Verification items for the finished model (mm, model axes). Face numbers are marked on the shaded views. A direction names the side the tool comes from. Coordinates: 2 decimals unless noted, no trailing zeros. Loops run counter-clockwise (first coordinate to the right, second up) from the corner with the lowest first, then second, coordinate; pieces in that order, holes last. Notation, with made-up numbers: (-29.75, 50.25) -> (16.25, 50.25) arc R29 ccw to (16.25, 74.25) -> close; hole circle Ø9 at (23.25, 43). An arc over 180 degrees is marked (long way). Use CSV: the item, a comma, the result in double quotes. Start each with the question number.
Autodesk Inventor part; units mm, degrees
ref_plane "YZ Plane" through (0, 0, 0) normal (1, 0, 0) x (0, 1, 0)
ref_plane "XZ Plane" through (0, 0, 0) normal (0, 1, 0) x (-1, 0, 0)
ref_plane "XY Plane" through (0, 0, 0) normal (0, 0, 1) x (1, 0, 0)
sketch "スケッチ1" plane through (0, 0, 0) normal (1, 0, 0) x (0, 1, 0)
  circle A0 centre (0, 0) radius 10
  circle A1 centre (0, -10) radius 1.35
  circle A2 centre (8.6603, 5) radius 1.35
  circle A3 centre (-8.6603, 5) radius 1.35
  circle A4 centre (0, 0) radius 5
  line L0 (0, 0) -> (0, 50)
  circle A5 centre (0, 50) radius 22.5
  circle A6 centre (0, 0) radius 14
  line L1 (-14, 0) -> (-22.5, 50)
  line L2 (14, 0) -> (22.5, 50)
  line L3 (0, -14) -> (-11.62, -14)
  line L4 (-11.62, -14) -> (-14, 0)
  line L5 (0, -14) -> (11.62, -14)
  line L6 (11.62, -14) -> (14, 0)
  line L7 (0, 20) -> (-17.4, 20)
  line L8 (0, 20) -> (17.4, 20)
  dimension "d0" = 20
  dimension "d1" = 2.7
  dimension "d4" = 360
  dimension "d6" = 10
  dimension "d7" = 50
  dimension "d8" = 45
  dimension "d9" = 28
extrude "押し出し1" add sketch "スケッチ1" along normal blind 4 contours A0 A1 A3 A2 | A6 L6 L4 | A6 L1 L7 L0 | L0 L8 L2 A6 | L6 L5 A6 | A6 L3 L4
sketch "スケッチ2" plane through (0, -17.4, 20) normal (0, 0, 1) x (1, 0, 0)
  line L0 (0, 17.4) -> (30, 17.4)
  circle A0 centre (30, 17.4) radius 22.5
  circle A1 centre (30, 17.4) radius 18.5
  circle A2 centre (30, 17.4) radius 14
  circle A3 centre (48.5, 17.4) radius 1.35
  circle A4 centre (20.75, 33.4215) radius 1.35
  circle A5 centre (20.75, 1.3785) radius 1.35
  line L1 (0, 29.02) -> (0, 34.8)
  line L2 (0, 0) -> (0, 5.78)
  line L3 (0, 34.8) -> (0, 0)
  line L4 (4, 29.02) -> (4, 34.8)
  line L5 (4, 34.8) -> (7, 34.8)
  line L6 (7, 34.8) -> (30, 39.9)
  line L7 (4, 0) -> (4, 5.78)
  line L8 (4, 0) -> (7, 0)
  line L9 (7, 0) -> (30, -5.1)
  line L10 (4, 0) -> (0, 0)
  line L11 (0, 34.8) -> (4, 34.8)
  line L12 (0, 0) -> (0, 34.8)
  line L13 (0, 34.8) -> (4, 34.8)
  dimension "d14" = 37
  dimension "d12" = 30
  dimension "d13" = 45
  dimension "d15" = 28
  dimension "d16" = 2.7
  dimension "d19" = 360
  dimension "d21" = 3
  dimension "d22" = 3
extrude "押し出し2" add sketch "スケッチ2" along normal blind 4 contours L3 L1 L11 L5 L6 A0 L0 | L0 A0 L9 L8 L10 L2 L3 | A1 A4 A3 A5 | A0 L6 L9
fillet "フィレット1" radius 3 2 edges at (4, 0, 20) (0, 0, 24)
fillet "フィレット2" radius 3 2 edges at (2, -11.62, -14) (2, 11.62, -14)
sketch "スケッチ7" plane through (0, -17.4, 24) normal (0, 0, 1) x (1, 0, 0)
  circle A0 centre (30, 17.4) radius 14
  line L0 (30, 17.4) -> (182.95, 17.4)
  line L1 (30, 17.4) -> (182.95, 17.4) construction
  circle A1 centre (182.95, 17.4) radius 3.5
  circle A2 centre (182.95, 17.4) radius 10
  line L2 (182.95, 27.4) -> (50.1556, 27.4)
  arc A3 (30, -5.1) -> (30, 39.9) centre (30, 17.4) ccw
  line L3 (182.95, 27.4) -> (315.7444, 27.4) construction
  line L4 (182.95, 7.4) -> (50.1556, 7.4)
  point P0 (0, 17.4)
  dimension "d55" = 152.95
  dimension "d56" = 0
  dimension "d57" = 7
  dimension "d58" = 20
  dimension "d59" = 180
extrude "押し出し7" add sketch "スケッチ7" against normal blind 4 contours A3 L2 A2 L0 | L0 A2 L4 A3 | A2
fillet "フィレット3" radius 2 2 edges at (50.1556, 10, 22) (50.1556, -10, 22)
sketch "スケッチ8" plane through (0, -17.4, 24) normal (0, 0, 1) x (1, 0, 0)
  circle A0 centre (20.75, 33.4215) radius 1.35
  circle A1 centre (20.75, 33.4215) radius 2.5
  circle A2 centre (48.5, 17.4) radius 1.35
  circle A3 centre (48.5, 17.4) radius 2.5
  circle A4 centre (20.75, 1.3785) radius 1.35
  circle A5 centre (20.75, 1.3785) radius 2.5
  point P0 (0, 17.4)
  dimension "d63" = 5
  dimension "d64" = 5
  dimension "d65" = 5
extrude "押し出し8" cut sketch "スケッチ8" against normal blind 2 contours A0 | A1 | A3 | A4 | A5
properties part number "motor_holder_2" material "アルミニウム 6061"
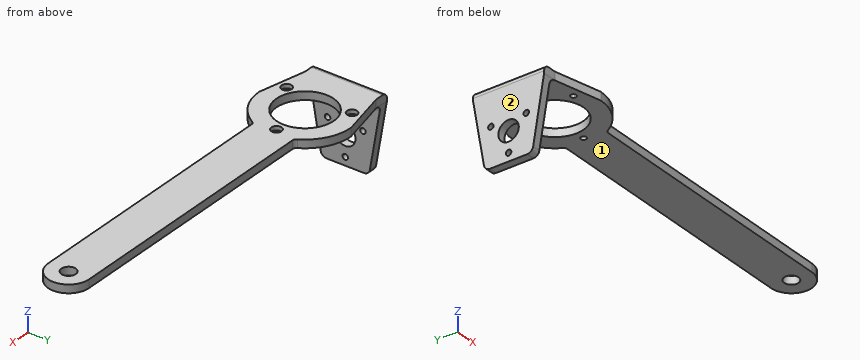
1. Cross-section at B-B, the plane z = 9. Record the boundary of the cut face in (x, y), plus the area to 3 significant figures.
2. Cross-section at A-A, the plane x = 73. Record the boundary of the cut face in (y, z), plus the area to 3 significant figures.
3. Set-up check for the marked faces 1 and 2: record each of +Z, -Z, +X, -X, +Y, -Y from which the full face is reachable in a straight line by a thin tool's end or side.
4. Scan lines: line 1 (Z direction, x = 2.6, y = 0); line 2 (Y direction, x = 30, z = 21.1); line 3 (Y direction, x = 20.75, z = 23.2). Record each from-to range of solid material in increasing order.
5. Depth check by flat-ended pin: pin 1 (6 mm diameter, centred on y = 9.5, z = 4, fed in from +X); pin 2 (13.5 mm diameter, centred on x = 59.5, y = -1, fed in from -Z); pin 3 (3 mm diameter, centred on x = 3.5, z = 22, fed in from -Y). Enter the tip coordinate at first touch or a pass-through.
Solution:
1,outline,"(0, -15.53) -> (4, -15.53) -> (4, 15.53) -> (0, 15.53) -> close"
1,area,"124 mm2"
2,outline,"(-10, 20) -> (10, 20) -> (10, 24) -> (-10, 24) -> close"
2,area,"80.0 mm2"
3,face 1,"-Z, +X, +Y, -Y"
3,face 2,"+Z, -Z, -X, +Y, -Y"
4,line 1,"z = -14 to -11.35, -8.65 to -5, 5 to 23.97"
4,line 2,"y = -22.5 to -14, 14 to 22.5"
4,line 3,"y = -20.45 to -18.52, -13.52 to -10.51, 10.51 to 13.52, 18.52 to 20.45"
5,pin 1,"stops at x = 4"
5,pin 2,"stops at z = 20"
5,pin 3,"stops at y = -17.4"
